Geometry check sheet. Reference: the model listing, model coordinates, mm. Face numbers are marked on the shaded views. A direction names the side the tool comes from. Coordinates: 2 decimals unless noted, no trailing zeros. Order: outer loops, then holes, each group sorted by start corner. A loop starts at its lowest first (then second) coordinate and runs counter-clockwise, first axis right, second up. Notation, with made-up numbers: (50, 69.5) - (109, 69.5) arc R23 ccw to (109, 80.5) - close; hole circle Ø5 at (26.25, 1.5). An arc over 180 degrees is marked (long way). Return JSON: item names as keys, results as strings. Group by question number.
Item 1: Section check C-C on x = -6. Enter the section's corners in (y, z).
Item 2: Section check D-D on z = -4.75. Enter the section's corners in (x, y).
Item 3: Draft check along Z on the marked faces 3, 4 and 5. Enter one of: pulls with the +Z half, pulls with the -Z half, needs draft (parallel to the pull), parting line crosses it, or undercut.
Item 4: Tool access check on the marked faces 1 and 2. Record the directions out of +Z, -Z, +X, -X, +Y, -Y that give a thin tool (end or side, any length) a straight path to the whole face; none if there is none.
Item 5: Section check B-B on x = 0. Enter the section's corners in (y, z), then the cut area to 3 significant figures.
Item 6: Gauge pin test, flat ends, axial feed: pin 1 (3 mm diameter, centred on x = -0.5, z = 0, fed in from +Y); pin 2 (6 mm diameter, centred on x = -4, z = 2, fed in from +Y); pin 3 (2.5 mm diameter, centred on x = 5, z = -5, fed in from -Y); pin 4 (4 mm diameter, centred on y = 1.5, z = 7.5, fed in from -X). Record the tip position at first contact, or that the pin passes through.
Item 7: Scan lines: probe 1 along X at (y, z) = (1.85, -5); probe 2 along X at (y, z) = (2, 3.75); probe 3 along Z at (x, y) = (-5.5, 1.5). Record each from-to range of solid material in increasing order.
Item 8: Section check A-A on z = 0. Enter the section's corners in (x, y).
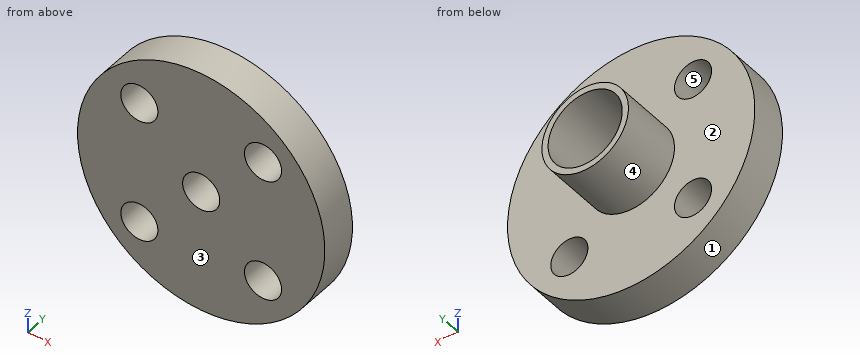
from build123d import *

# Parameters (mm, degrees)
SKETCH_1_R          = 10
SKETCH_1_R_2        = 1.5
EXTRUDE_1_DEPTH     = 3
SKETCH_2_R          = 3.5
SKETCH_2_R_2        = 3
EXTRUDE_2_DEPTH     = 5
SKETCH_3_R          = 1.5
CUT_EXTRUDE_1_DEPTH = 5


with BuildPart() as part:
    # 草图1 → 凸台-拉伸1 (new body)
    with BuildSketch(Plane(origin=(0, 0, 0), x_dir=(1, 0, 0), z_dir=(0, 1, 0))):
        with Locations(Location((0, 0, 0), (0, 0, 270))):
            Circle(SKETCH_1_R)
        with Locations(Location((-5, 5, 0), (0, 0, 270))):
            Circle(SKETCH_1_R_2, mode=Mode.SUBTRACT)
        with Locations(Location((5, 5, 0), (0, 0, 270))):
            Circle(SKETCH_1_R_2, mode=Mode.SUBTRACT)
        with Locations(Location((5, -5, 0), (0, 0, 270))):
            Circle(SKETCH_1_R_2, mode=Mode.SUBTRACT)
        with Locations(Location((-5, -5, 0), (0, 0, 270))):
            Circle(SKETCH_1_R_2, mode=Mode.SUBTRACT)
    extrude(amount=EXTRUDE_1_DEPTH)

    # 草图2 → 凸台-拉伸2 (add)
    with BuildSketch(Plane(origin=(0, 3, 0), x_dir=(1, 0, 0), z_dir=(0, 1, 0))):
        with Locations(Location((0, 0, 0), (0, 0, 270))):
            Circle(SKETCH_2_R)
        with Locations(Location((0, 0, 0), (0, 0, 270))):
            Circle(SKETCH_2_R_2, mode=Mode.SUBTRACT)
    extrude(amount=EXTRUDE_2_DEPTH)

    # 草图3 → 切除-拉伸1 (cut)
    with BuildSketch(Plane(origin=(0, 3, 0), x_dir=(1, 0, 0), z_dir=(0, 1, 0))):
        with Locations(Location((0, 0, 0), (0, 0, 270))):
            Circle(SKETCH_3_R)
    extrude(amount=-CUT_EXTRUDE_1_DEPTH, mode=Mode.SUBTRACT)


solid = part.part
Computed:
{
 "1": {"outline": "(0, -8) - (3, -8) - (3, -6.12) - (0, -6.12) - close; (0, -3.88) - (3, -3.88) - (3, 3.88) - (0, 3.88) - close; (0, 6.12) - (3, 6.12) - (3, 8) - (0, 8) - close"},
 "2": {"outline": "(-8.8, 0) - (-6.48, 0) - (-6.48, 3) - (-8.8, 3) - close; (-3.52, 0) - (3.52, 0) - (3.52, 3) - (-3.52, 3) - close; (6.48, 0) - (8.8, 0) - (8.8, 3) - (6.48, 3) - close"},
 "3": {"face 3": "needs draft", "face 4": "parting line crosses it", "face 5": "undercut"},
 "4": {"face 1": "+Y, -Y", "face 2": "+Y"},
 "5": {"outline": "(0, -10) - (3, -10) - (3, -3.5) - (8, -3.5) - (8, -3) - (3, -3) - (3, -1.5) - (0, -1.5) - close; (0, 1.5) - (3, 1.5) - (3, 3) - (8, 3) - (8, 3.5) - (3, 3.5) - (3, 10) - (0, 10) - close", "area": "56.0 mm²"},
 "6": {"pin 1": "stops at y = 3", "pin 2": "stops at y = 8", "pin 3": "passes through", "pin 4": "stops at x = -8.35"},
 "7": {"probe 1": "x = -8.66 to -6.5, -3.5 to 3.5, 6.5 to 8.66", "probe 2": "x = -9.27 to -5.83, -4.17 to 4.17, 5.83 to 9.27", "probe 3": "z = -8.35 to -6.41, -3.59 to 3.59, 6.41 to 8.35"},
 "8": {"outline": "(-10, 0) - (-1.5, 0) - (-1.5, 3) - (-3, 3) - (-3, 8) - (-3.5, 8) - (-3.5, 3) - (-10, 3) - close; (1.5, 0) - (10, 0) - (10, 3) - (3.5, 3) - (3.5, 8) - (3, 8) - (3, 3) - (1.5, 3) - close"}
}
